Autodesk Inventor part; units mm, degrees
ref_plane "YZ Plane" through (0, 0, 0) normal (1, 0, 0) x (0, 1, 0)
ref_plane "XZ Plane" through (0, 0, 0) normal (0, 1, 0) x (-1, 0, 0)
ref_plane "XY Plane" through (0, 0, 0) normal (0, 0, 1) x (1, 0, 0)
sketch "Sketch3" plane through (0, 0, 0) normal (0, 0, 1) x (1, 0, 0)
  circle A0 centre (0, 0) radius 22.5
  line L0 (-8.5, 0) -> (8.5, 0)
  line L1 (8.5, 0) -> (8.5, 83)
  line L2 (8.5, 83) -> (-8.5, 83)
  line L3 (-8.5, 83) -> (-8.5, 0)
  dimension "d5" = 45
  dimension "d6" = 83
  dimension "d7" = 17
extrude "Extrusion3" add sketch "Sketch3" along normal blind 15
sketch "Sketch4" plane through (0, 0, 0) normal (0, 0, -1) x (-1, 0, 0)
  arc A0 (-8.5, 20.8327) -> (8.5, 20.8327) centre (0, 0) ccw
  line L0 (8.5, 83) -> (8.5, 20.8327)
  line L1 (-8.5, 83) -> (8.5, 83)
  line L2 (-8.5, 20.8327) -> (-8.5, 83)
  arc A1 (-6.5, 19.4422) -> (6.5, 19.4422) centre (0, 0) ccw
  line L3 (-6.5, 19.4422) -> (-6.5, 81)
  line L4 (-6.5, 81) -> (6.5, 81)
  line L5 (6.5, 81) -> (6.5, 19.4422)
  dimension "d10" = 2
extrude "Extrusion4" cut sketch "Sketch4" against normal blind 13 contours L3 L4 L5 A1
chamfer "Chamfer1" distance 5 angle 45 1 edges at (0, 83, 15)
sketch "Sketch6" plane through (-8.5, 78, 15) normal (0, 0.7071068, 0.7071068) x (1, 0, 0)
  line L0 (2, 2.8284) -> (2, 4.2426)
  line L1 (2, 4.2426) -> (15, 4.2426)
  line L2 (15, 4.2426) -> (15, 2.8284)
  line L3 (15, 2.8284) -> (2, 2.8284)
  line L4 (0, 7.0711) -> (0, 0)
  line L5 (0, 0) -> (17, 0)
  line L6 (17, 0) -> (17, 7.0711)
  line L7 (17, 7.0711) -> (0, 7.0711)
  point P0 (8.5, -44.5477)
extrude "Extrusion5" add sketch "Sketch6" against normal blind 2 contours L0 L1 L2 L3 | L7 L6 L5 L4
properties part number "TARM10" material "ABS Plastic"
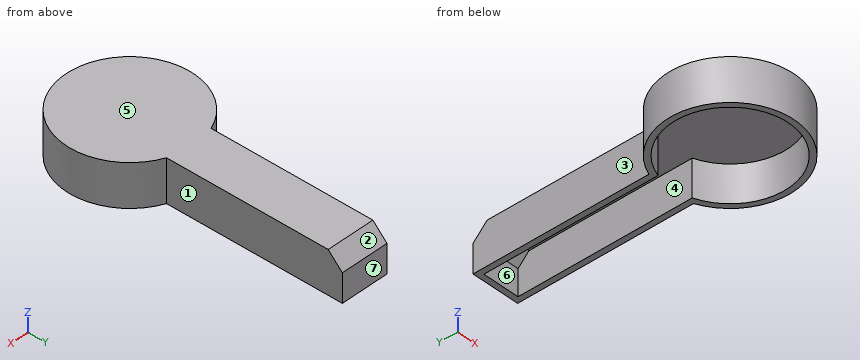
Design review of the part built by this model. Coordinates are the model's own, in mm. Face numbers are marked on the shaded views. A direction names the side the tool comes from. Give positions to 0.01 mm unless a question says otherwise; leave off trailing zeros. Loops run counter-clockwise (first coordinate to the right, second up) from the corner with the lowest first, then second, coordinate; pieces in that order, holes last. Notation, with made-up numbers: M 15.25,28.5 L 32.25,28.5 A22 cw 32.25,44.5 Z; hole C -36.5,12.25 d2. An arc over 180 degrees is marked long. Answer as a JSON object with one key per item and string values.
Item 1: Mouldability with a two-part tool opening along Y and no side actions: class the marked faces 5, 6 and 7 as pulls with the +Y half, pulls with the -Y half, needs draft (parallel to the pull), parting line crosses it, or undercut.
Output values:
{"face 5": "needs draft", "face 6": "undercut", "face 7": "pulls with the +Y half"}
Item 2: We need section A-A (z = 7). State the section outline as (x, y) points, and give its area (3 significant figures).
Output values:
{"outline": "M -8.5,20.83 A22.5 ccw long 8.5,20.83 L 8.5,83 L -8.5,83 Z; hole M -6.5,19.44 A20.5 ccw long 6.5,19.44 L 6.5,81 L -6.5,81 Z", "area": "517 mm2"}
Item 3: We need section D-D (z = 11.75). State the section outline as (x, y) points, and give its area (3 significant figures).
Output values:
{"outline": "M -8.5,20.83 A22.5 ccw long 8.5,20.83 L 8.5,81.25 L -8.5,81.25 Z; hole M -6.5,19.44 A20.5 ccw long 6.5,19.44 L 6.5,78.42 L -6.5,78.42 Z", "area": "521 mm2"}
Item 4: For P1, Ø4, axis at y = 11.5, z = 2, coming from the -X side; P2, Ø6.5, axis at y = 50, z = 8.5, coming from the +X side; P3, Ø5, axis at y = 29.5, z = 1.5, coming from the -X side, all flat-tipped, find the tip position at first contact; note any pin that passes through.
Output values:
{"P1": "stops at x = -20.4", "P2": "stops at x = 8.5", "P3": "stops at x = -8.5"}
Item 5: Machinability: for the marked faces 1, 2, 3 and 4, which of the approach directions +Z, -Z, +X, -X, +Y, -Y give a long, thin tool a straight path to every point of the face, cutting with its end or side? Answer none if there is none.
Output values:
{"face 1": "+Z, -Z, +X, +Y", "face 2": "+Z, +X, -X, +Y", "face 3": "+Z, -Z, -X, +Y", "face 4": "-Z"}
Item 6: We need section B-B (x = 0). State the section outline as (y, z) points, and give its area (3 significant figures).
Output values:
{"outline": "M -22.5,0 L -20.5,0 L -20.5,13 L 77.17,13 L 81,9.17 L 81,0 L 83,0 L 83,10 L 78,15 L -22.5,15 Z", "area": "258 mm2"}
Item 7: Wall thickness on line 1 along Y through (x, z) = (0, 3.75); line 2 along X through (y, z) = (51, 6); line 3 along X through (y, z) = (0, 3.25): over which ranges is each line inside the solid? List them lowest first.
Output values:
{"line 1": "y = -22.5 to -20.5, 81 to 83", "line 2": "x = -8.5 to -6.5, 6.5 to 8.5", "line 3": "x = -22.5 to -20.5, 20.5 to 22.5"}
Item 8: We need section C-C (y = 42.5). State the section outline as (x, z) points, and give its area (3 significant figures).
Output values:
{"outline": "M -8.5,0 L -6.5,0 L -6.5,13 L 6.5,13 L 6.5,0 L 8.5,0 L 8.5,15 L -8.5,15 Z", "area": "86.0 mm2"}
